Could you check a few things on this model? Use its own coordinates, in mm. Face numbers are marked on the shaded views. A direction names the side the tool comes from. Give positions to 0.01 mm unless a question says otherwise; leave off trailing zeros. Order: outer loops, then holes, each group sorted by start corner. A loop starts at its lowest first (then second) coordinate and runs counter-clockwise, first axis right, second up. Notation, with made-up numbers: (76.25, -34.75) - (108.25, -34.75) arc R18 ccw to (108.25, -14.75) - close; hole circle Ø9 at (3, -21). An arc over 180 degrees is marked (long way). One line per question, with ' | ' between items. Start each with the question number.
1. For P1, Ø1.5, axis at x = -12.5, z = 1.5, coming from the -Y side; P2, Ø8, axis at x = -15, y = 0, coming from the +Z side; P3, Ø1.5, axis at y = -18, z = 3, coming from the -X side, each with a flat end and sliding along its axis, tell me the tip position at first contact or that it passes through.
2. If we mould it in two halves opening along X, with no side actions, what happens to the marked faces 5, 6 and 7? For each: released by +X, released by -X, zero draft, split by the parting line, or undercut.
3. Imagine slicing it at B-B (x = 0). Please give me the cut outline in (y, z).
4. Which directions (+Z, -Z, +X, -X, +Y, -Y) give clear straight access to the entire face, cutting with the end or side of a thin tool? Please do the marked faces 1, 2, 3 and 4.
5. Imagine slicing it at A-A (z = 3.75). Please give me the cut outline in (x, y), and give its area (3 significant figures).
6. I need wall thicknesses on probe 1 along Z at (x, y) = (-28, -9.5); probe 2 along Y at (x, z) = (0, 0.5); probe 3 along X at (y, z) = (-6, 4.5). Which ranges of each line are inside material? Lowest first, please. Write a range as from..to.
7. Imagine slicing it at C-C (y = -18). Please give me the cut outline in (x, z).
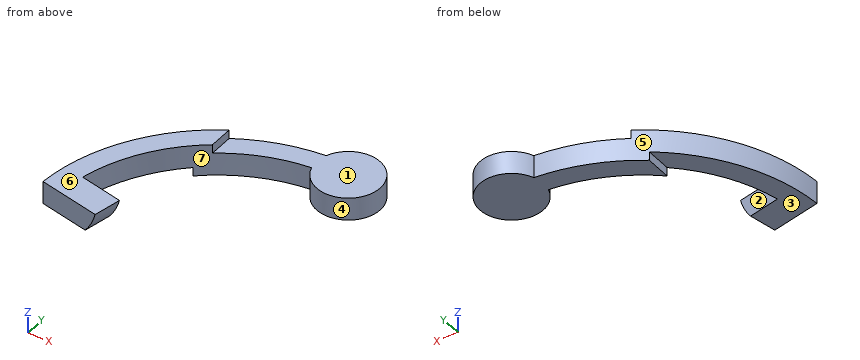
```python
from build123d import *

# Parameters (mm, degrees)
ESQUISSE3_R                  = 7
BOSS_EXTRU_2_DEPTH           = 5
BOSS_EXTRU_3_DEPTH           = 45
ENL_V_MAT_EXTRU_3_DEPTH      = 5
ENL_V_MAT_EXTRU_3_DEPTH_BACK = 73.880031702
ESQUISSE4_4_W                = 16.307493561
ESQUISSE4_4_H                = 1.918484986
ENL_V_MAT_EXTRU_4_DEPTH      = 58.743956008
ENL_V_MAT_EXTRU_6_DEPTH      = 57.375584133


with BuildPart() as part:
    # Esquisse3 → Boss.-Extru.2 (new body)
    with BuildSketch(Plane.XY):
        Circle(ESQUISSE3_R)
    extrude(amount=BOSS_EXTRU_2_DEPTH)

    # Esquisse3_3 → Boss.-Extru.3 (add)
    with BuildSketch(Plane.XY):
        with BuildLine():
            ThreePointArc((-6.556240583, 2.452694319), (-31.795381091, -9.503990443), (-43.059714875, -35.059641647))
            Line((-43.059714875, -35.059641647), (-29.67043681, -37.846531887))
            Line((-29.67043681, -37.846531887), (-28.42882324, -31.881349224))
            Line((-28.42882324, -31.881349224), (-37.880972605, -29.913946449))
            ThreePointArc((-37.880972605, -29.913946449), (-26.825365644, -10.900303142), (-6.699170831, -2.030051767))
            ThreePointArc((-6.699170831, -2.030051767), (-6.99644453, 0.22307834), (-6.556240583, 2.452694319))
        make_face()
    extrude(amount=BOSS_EXTRU_3_DEPTH)

    # Esquisse4 → Enl_v. mat.-Extru.3 (cut, two sides: drawn at the far end of the back side and taken through both)
    with BuildSketch(Plane(origin=(0, 0, 0), x_dir=(1, 0, 0), z_dir=(0, 1, 0)).offset(-ENL_V_MAT_EXTRU_3_DEPTH_BACK)):
        Polygon((-6.556240583, -21.643777245), (-6.556240583, -5), (-23.967427217, -5), (-23.967427217, -6.918484986), (-43.059714875, -6.918484986), (-43.059714875, -11.918484986), (-43.059714875, -45), (-43.059714875, -53.527020644), (-6.425184121, -53.527020644), align=None)
    extrude(amount=ENL_V_MAT_EXTRU_3_DEPTH + ENL_V_MAT_EXTRU_3_DEPTH_BACK, mode=Mode.SUBTRACT)

    # Esquisse4_4 → Enl_v. mat.-Extru.4 (cut, through all)
    with BuildSketch(Plane(origin=(0, 0, 0), x_dir=(1, 0, 0), z_dir=(0, 1, 0))):
        with Locations((-34.905968095, -0.959242493)):
            Rectangle(ESQUISSE4_4_W, ESQUISSE4_4_H)
    extrude(amount=-ENL_V_MAT_EXTRU_4_DEPTH, mode=Mode.SUBTRACT)

    # Esquisse5 → Enl_v. mat.-Extru.6 (cut, through all)
    with BuildSketch(Plane(origin=(-7.540837864, -36.229046112, 0), x_dir=(0.9790175257089632, -0.2037760642340011, 0), z_dir=(0.2037760642340011, 0.9790175257089632, 0))):
        with BuildLine():
            Line((-23.948753957, -1.918484986), (-21.33566032, -1.918484986))
            Line((-21.33566032, -1.918484986), (-21.33566032, -6.918484986))
            ThreePointArc((-21.33566032, -6.918484986), (-22.389352617, -4.286338478), (-23.948753957, -1.918484986))
        make_face()
    extrude(amount=-ENL_V_MAT_EXTRU_6_DEPTH, mode=Mode.SUBTRACT)


solid = part.part
```
Results found:
1) P1: stops at y = -3.32 | P2: stops at z = 5 | P3: stops at x = -38.51
2) face 5: released by -X | face 6: zero draft | face 7: undercut
3) outline: (-7, 0) - (7, 0) - (7, 5) - (-7, 5) - close
4) face 1: +Z, +X, +Y, -Y | face 2: +Z, -Z, +X | face 3: -Z, -X, +Y, -Y | face 4: +Z, -Z
5) outline: (-43.06, -35.06) - (-30.99, -37.57) - (-29.75, -31.61) - (-37.88, -29.91) arc R35.55 cw to (-6.7, -2.03) arc R7 ccw (long way) to (-6.56, 2.45) arc R40 ccw to start | area: 443 mm2
6) probe 1: z = 1.92..6.92 | probe 2: y = -7..7 | probe 3: x = -27.91..-19.8, -3.61..3.61
7) outline: (-38.11, 1.92) - (-32.92, 1.92) - (-32.92, 6.92) - (-38.11, 6.92) - close
